Autodesk Inventor part; units mm, degrees
ref_plane "Work Plane1" through (2.5, 6.5, 33) normal (0, -1, 0) x (1, 0, 0)
ref_plane "YZ Plane" through (0, 0, 0) normal (1, 0, 0) x (0, 1, 0)
ref_plane "XZ Plane" through (0, 0, 0) normal (0, 1, 0) x (-1, 0, 0)
sketch "Sketch1" plane through (0, 0, 0) normal (0, 0, 1) x (1, 0, 0)
  line L0 (0, 17.6) -> (0, -13.2)
  line L1 (-2.5, 0) -> (32.5, 0)
  line L2 (0, 11) -> (25, 11)
  line L3 (25, 11) -> (25, -11)
  line L4 (25, -11) -> (0, -11)
  line L5 (0, -11) -> (0, 11)
  dimension "d0" = 22
  dimension "d1" = 25
extrude "Extrusion1" add sketch "Sketch1" along normal blind 35
sketch "Sketch2" plane through (0, -11, 0) normal (-1, 0, 0) x (0, 0, 1)
  line L0 (0, 0) -> (0, 22)
  line L1 (-3.5, 11) -> (45.5, 11)
  line L2 (4, 18.5) -> (10, 18.5)
  line L3 (10, 18.5) -> (10, 3.5)
  line L4 (10, 3.5) -> (4, 3.5)
  line L5 (4, 3.5) -> (4, 18.5)
  line L6 (12.5, 18.5) -> (18.5, 18.5)
  line L7 (18.5, 18.5) -> (18.5, 3.5)
  line L8 (18.5, 3.5) -> (12.5, 3.5)
  line L9 (12.5, 3.5) -> (12.5, 18.5)
  line L10 (20.5, 18.5) -> (27.5, 18.5)
  line L11 (27.5, 18.5) -> (27.5, 3.5)
  line L12 (27.5, 3.5) -> (20.5, 3.5)
  line L13 (20.5, 3.5) -> (20.5, 18.5)
  line L14 (27.5, 17) -> (31.5, 17)
  line L15 (31.5, 17) -> (31.5, 5)
  line L16 (31.5, 5) -> (27.5, 5)
  line L17 (27.5, 5) -> (27.5, 17)
  dimension "d4" = 4
  dimension "d5" = 15
  dimension "d6" = 2.5
  dimension "d7" = 6
  dimension "d8" = 11
  dimension "d9" = 2
  dimension "d10" = 7
  dimension "d11" = 12
extrude "Extrusion2" cut sketch "Sketch2" against normal blind 20
sketch "Sketch3" plane through (20, -11, 0) normal (-1, 0, 0) x (0, 0, 1)
  line L0 (10, 3.5) -> (10, 18.5)
  line L1 (9, 18) -> (7.5, 18)
  line L2 (7.5, 18) -> (7.5, 4)
  line L3 (7.5, 4) -> (9, 4)
  line L4 (9, 4) -> (9, 18)
  line L5 (17.5, 18) -> (16, 18)
  line L6 (16, 18) -> (16, 4)
  line L7 (16, 4) -> (17.5, 4)
  line L8 (17.5, 4) -> (17.5, 18)
  line L9 (12.5, 18.5) -> (12.5, 3.5)
  line L10 (12.5, 3.5) -> (18.5, 3.5)
  line L11 (18.5, 3.5) -> (18.5, 18.5)
  line L12 (18.5, 18.5) -> (12.5, 18.5)
  line L13 (-3.5, 11) -> (45.5, 11)
  dimension "d14" = 1.5
  dimension "d15" = 1
  dimension "d16" = 1
  dimension "d17" = 14
extrude "Extrusion3" add sketch "Sketch3" along normal blind 18 contours L4 L13 L2 L1 | L4 L3 L2 L13 | L13 L8 L7 L6 | L6 L5 L8 L13
sketch "Sketch4" plane through (0, 0, 0) normal (0, 1, 0) x (-1, 0, 0)
  line L0 (-20, 27.5) -> (-20, 20.5)
  line L1 (0, 20.5) -> (-20, 20.5)
  line L2 (-20, 23) -> (-2, 20.5)
  line L3 (0, 0) -> (0, 35)
  dimension "d20" = 2
  dimension "d21" = 2.5
extrude "Extrusion4" add sketch "Sketch4" along normal mid plane 10
sketch "Sketch5" plane through (20, -11, 0) normal (-1, 0, 0) x (0, 0, 1)
  line L0 (20.5, 16) -> (23, 16)
  line L1 (23, 16) -> (23, 6)
  line L2 (20.5, 3.5) -> (20.5, 18.5)
  line L3 (20.5, 15.8) -> (23, 15.8)
  line L4 (23, 15.8) -> (23, 15.3)
  line L5 (23, 15.3) -> (20.5, 15.3)
  line L6 (20.5, 15.3) -> (20.5, 15.8)
  dimension "d24" = 0.2
  dimension "d25" = 0.5
extrude "Extrusion5" cut sketch "Sketch5" along normal through all contours L3 L1 L5 L2
pattern_linear "Rectangular Pattern1" count 14 spacing 0.7 along (0, -1, 0) of "Extrusion5"
sketch "Sketch6" plane through (0, 0, 35) normal (0, 0, 1) x (1, 0, 0)
  line L0 (0, 11) -> (25, 11)
  line L1 (0, -11) -> (0, 11)
  line L2 (2.5, 8.5) -> (14.5, 8.5)
  line L3 (14.5, 8.5) -> (14.5, 4.5)
  line L4 (14.5, 4.5) -> (2.5, 4.5)
  line L5 (2.5, 4.5) -> (2.5, 8.5)
  dimension "d31" = 2.5
  dimension "d32" = 12
  dimension "d33" = 4
  dimension "d34" = 2.5
extrude "Extrusion6" cut sketch "Sketch6" against normal blind 2
ref_plane "Work Plane1" through (2.5, 6.5, 33) normal (0, -1, 0) x (1, 0, 0)
sketch "Sketch7" plane through (2.5, 6.5, 33) normal (0, -1, 0) x (1, 0, 0)
  line L0 (0, 2) -> (0, 0) construction
  line L1 (0, 2) -> (3.0475, 2.2666)
  line L2 (8.95, 2.2854) -> (11, 3.2413)
  arc A0 (8.95, 2.2854) -> (3.0475, 2.2666) centre (6.0291, -7.2785) ccw
  line L3 (0, 1.7992) -> (3.0866, 2.0693)
  arc A1 (8.9646, 2.0715) -> (3.0866, 2.0693) centre (6.0291, -7.2785) ccw
  line L4 (8.9646, 2.0715) -> (11.0845, 3.06)
  line L5 (11, 3.2413) -> (11.0845, 3.06)
  line L6 (0, 2) -> (0, 1.7992)
  dimension "d37" = 11
  dimension "d38" = 95
  dimension "d39" = 10
  dimension "d40" = 65
  dimension "d41" = 0.2
extrude "Extrusion7" add sketch "Sketch7" along normal mid plane 3.5
mirror "Mirror1" about plane through (0, 0, 0) normal (0, 1, 0) of "Extrusion6", "Extrusion7"
equation "\"d16\" = d15"
properties part number "config - nic module"
Build history of the part. All positions in model axes, mm. A direction names the side the tool comes from. Round coordinates to 2 decimals unless told otherwise and drop trailing zeros. Write each loop counter-clockwise with the first axis right and the second up, starting at its lowest first coordinate (ties: lowest second). Pieces come first, ordered by that corner, then holes. Notation, with made-up numbers: M -36,49.25 L -5,49.25 A11 ccw -5,53.25 Z; hole C 75,22 d1. An arc over 180 degrees is marked long. Answer as a JSON object with one key per item and string values. Group by question number.
(1) Cut at A-A (z = 27). Give the cut face in (x, y), and give its area (3 significant figures).
(2) Mould opens along X. For faces 4 (the flat face through (8, -4.5, 34)), 5 (the flat face through (13, 2, 21)), 6 (the flat face through (12.51, 6.52, 35.56)) say: pulls with the +X half, pulls with the -X half, needs draft (parallel to the pull), parting line crosses it, or undercut.
(3) Cut at D-D (y = -9.5). Give the cut face in (x, z), and give its area (3 significant figures).
(4) Cut at B-B (x = 8.5). Give the number of separate pieces and of enclosed holes in the cut face, and give its area (3 significant figures).
(5) Cut at C-C (x = 20.5). Give the cut face in (y, z), and give its area (3 significant figures).
(6) Flat gauge pins, fed straight in: pin 1 (1 mm diameter, centred on x = 3, y = 0.5, fed in from +Z); pin 2 (1.5 mm diameter, centred on x = 18, y = -2.5, fed in from -Z); pin 3 (3 mm diameter, centred on y = 3.5, z = 7, fed in from -X). Where does each tip first touch, or does it go through?
(7) Which spindle directions (+Z, -Z, +X, -X, +Y, -Y) get a long thin tool onto all of the face, cutting with end or side? Do faces 1 (the flat face through (2.5, -7, 34)), 2 (the flat face through (14.5, 7, 34)), 3 (the flat face through (11, 7, 8)). Say none if no direction does.
(8) Drill centre lines: L1, parallel to Z at x = 4.25, y = 2.5; L2, parallel to Y at x = 13.5, z = 17; L3, parallel to Z at x = 3, y = 0.75. Where is each one in solid material? Low to high.
Responses:
{
 "1": {"outline": "M 0,-11 L 25,-11 L 25,11 L 0,11 L 0,7.5 L 20,7.5 L 20,-7.5 L 0,-7.5 Z", "area": "250 mm2"},
 "2": {"face 4": "undercut", "face 5": "needs draft", "face 6": "pulls with the +X half"},
 "3": {"outline": "M 0,0 L 25,0 L 25,35 L 0,35 Z", "area": "875 mm2"},
 "4": {"separate pieces": "5", "enclosed holes": "3", "area": "467 mm2"},
 "5": {"outline": "M -11,0 L 11,0 L 11,35 L -11,35 Z", "area": "770 mm2"},
 "6": {"pin 1": "stops at z = 35", "pin 2": "stops at z = 0", "pin 3": "stops at x = 2"},
 "7": {"face 1": "none", "face 2": "+Z", "face 3": "-X"},
 "8": {"L1": "z = 0 to 4, 7.5 to 9, 10 to 12.5, 16 to 17.5, 18.5 to 20.5, 31.5 to 35", "L2": "y = -11 to -7.5, -7 to 7, 7.5 to 11", "L3": "z = 0 to 4, 7.5 to 9, 10 to 12.5, 16 to 17.5, 18.5 to 20.64, 31.5 to 35"}
}
